from build123d import *

# Parameters (mm, degrees)
F0_W     = 50
F0_H     = 30
F1_DEPTH = 7
F2_R     = 5
F3_R     = 2


with BuildPart() as f1:
    # F0 (on Top) → F1 (new body)
    with BuildSketch(Plane.XY):
        Rectangle(F0_W, F0_H)
    extrude(amount=F1_DEPTH)

    # F2
    f2_edges = [f1.edges().sort_by_distance(p)[0] for p in [
        (25, -15, 3.5),
        (-25, -15, 3.5),
        (25, 15, 3.5),
        (-25, 15, 3.5),
    ]]
    fillet(f2_edges, radius=F2_R)

    # F3
    f3_edges = [f1.edges().sort_by_distance(p)[0] for p in [
        (0, -15, 7),
        (0, -15, 0),
    ]]
    fillet(f3_edges, radius=F3_R)


solid = f1.part
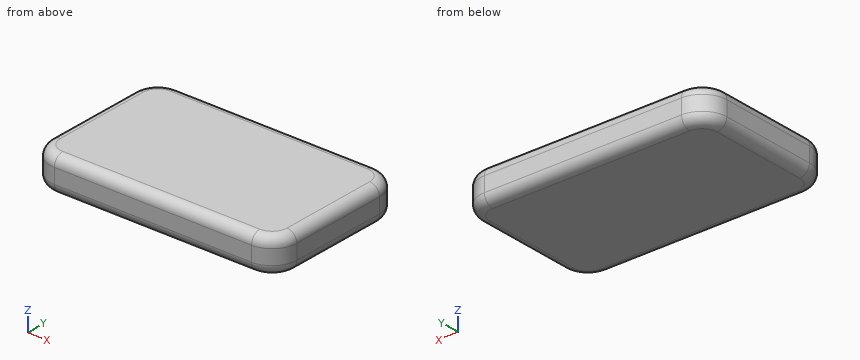
For this review, take the finished solid that the model builds, in its own axes (mm). Give positions to 0.01 mm unless a question says otherwise; leave off trailing zeros. Loops run counter-clockwise (first coordinate to the right, second up) from the corner with the lowest first, then second, coordinate; pieces in that order, holes last. Notation, with made-up numbers: M 49.25,-38 L 102.25,-38 A16 cw 102.25,-24 Z; hole C 62,12 d10. An arc over 180 degrees is marked long. Answer as a JSON object with one key per item and string values. Group by question number.
Q1. Add section B-B on z = 1.25. Give the boundary of the cut face in (x, y), and give its area (3 significant figures).
Q2. Add section A-A on x = -18. Give the boundary of the cut face in (y, z).
Q3. Insertion check: P1, Ø2, axis at y = 11.5, z = 1, coming from the -X side. The pin has a flat end and moves straight along its axis. Give the tip position at first contact, or say it passes through.
Q4. For probe 1 along Y at (x, z) = (-18, 5.5); probe 2 along X at (y, z) = (11, 1.25); probe 3 along X at (y, z) = (11.5, 2.75), list the stretches that pass through material, from the lowest coordinate up. Write a range as [from, to].
Checked values:
{
 "1": {"outline": "M -24.85,-10 A4.85 ccw -20,-14.85 L 20,-14.85 A4.85 ccw 24.85,-10 L 24.85,10 A4.85 ccw 20,14.85 L -20,14.85 A4.85 ccw -24.85,10 Z", "area": "1,460 mm²"},
 "2": {"outline": "M -15,2 A2 ccw -13,0 L 13,0 A2 ccw 15,2 L 15,5 A2 ccw 13,7 L -13,7 A2 ccw -15,5 Z"},
 "3": {"P1": "x = -24.91"},
 "4": {"probe 1": "[-14.94, 14.94]", "probe 2": "[-24.75, 24.75]", "probe 3": "[-24.77, 24.77]"}
}
